```python
from build123d import *

# Parameters (mm, degrees)
F0_W     = 120
F0_H     = 80
F1_DEPTH = 45
F2_R     = 8
F3_T     = -3
F5_DEPTH = 1.5


with BuildPart() as f1:
    # F0 (on Front) → F1 (new body, symmetric)
    with BuildSketch(Plane.XZ):
        Rectangle(F0_W, F0_H)
    extrude(amount=F1_DEPTH, both=True)

    # F2
    f2_edges = [f1.edges().sort_by_distance(p)[0] for p in [
        (60, 0, 40),
        (60, -45, 0),
        (60, 45, 0),
        (-60, 45, 0),
        (0, 45, 40),
        (-60, 0, 40),
        (-60, -45, 0),
        (0, -45, 40),
    ]]
    fillet(f2_edges, radius=F2_R)

    # F3
    f3_openings = [f1.faces().sort_by_distance(p)[0] for p in [
        (0, 0, -40),
    ]]
    offset(amount=F3_T, openings=f3_openings)

    # F4 (on face) → F5 (cut)
    with BuildSketch(Plane(origin=(0, 0, -40), x_dir=(1, 0, 0), z_dir=(0, 0, -1))):
        with BuildLine():
            Line((52, 43.2), (-52, 43.2))
            ThreePointArc((-52, 43.2), (-56.3840620434, 41.3840620434), (-58.2, 37))
            Line((-58.2, 37), (-58.2, -37))
            ThreePointArc((-58.2, -37), (-56.3840620434, -41.3840620434), (-52, -43.2))
            Line((-52, -43.2), (52, -43.2))
            ThreePointArc((52, -43.2), (56.3840620434, -41.3840620434), (58.2, -37))
            Line((58.2, -37), (58.2, 37))
            ThreePointArc((58.2, 37), (56.3840620434, 41.3840620434), (52, 43.2))
        make_face()
    extrude(amount=-F5_DEPTH, mode=Mode.SUBTRACT)


solid = f1.part
```
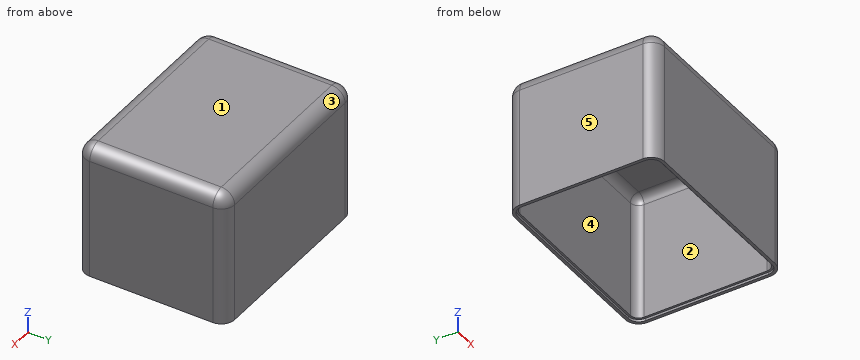
Read the model definition and answer for the solid it produces. Units are mm, in the model's axes. Face numbers are marked on the shaded views. A direction names the side the tool comes from. Give positions to 0.01 mm unless a question says otherwise; leave off trailing zeros. Write each loop counter-clockwise with the first axis right and the second up, starting at its lowest first coordinate (ties: lowest second). Pieces come first, ordered by that corner, then holes. Notation, with made-up numbers: M 23.5,51.25 L 40.5,51.25 A19 cw 40.5,65.25 Z; hole C -2.75,59.25 d6. An arc over 180 degrees is marked long. Put each result on its own line as item: value. Start each with the question number.
1. The part is cut by section B-B, the plane x = 32.5. Give the vertices of the cut face in (y, z), and give its area (3 significant figures).
2. Which of the six approach directions +Z, -Z, +X, -X, +Y, -Y give full straight-line access (tool end or side, diameter ignored) to the marked faces 4 and 5?
3. This flat-tipped pin is pushed along its axis until it touches: pin 1 Ø12 at (x, y) = (32, -23) entering from -Z. Where does it stop, or does it pass through?
4. For a pull along Y with two mould halves and no side action, classify the marked faces 1, 2 and 3 as released by +Y, released by -Y, zero draft, split by the parting line, or undercut.
5. Consider line 1 along Y through (x, z) = (-13.5, 9.5); line 2 along X through (y, z) = (-27.5, 24.5); line 3 along Z through (x, y) = (-51, 14). Determine where each line is inside the solid, lowest interval first.
6. The part is cut by section A-A, the plane z = -13. Give the vertices of the cut face in (x, y), and give its area (3 significant figures).
7. The part is cut by section C-C, the plane y = 25.5. Give the vertices of the cut face in (x, z), and give its area (3 significant figures).
Final values:
1. outline: M -45,-40 L -43.2,-40 L -43.2,-38.5 L -42,-38.5 L -42,32 A5 cw -37,37 L 37,37 A5 cw 42,32 L 42,-38.5 L 43.2,-38.5 L 43.2,-40 L 45,-40 L 45,32 A8 ccw 37,40 L -37,40 A8 ccw -45,32 Z
1. area: 712 mm²
2. face 4: -Z
2. face 5: +Z, -Z, -X, +Y, -Y
3. pin 1: stops at z = 37
4. face 1: zero draft
4. face 2: undercut
4. face 3: released by +Y
5. line 1: y = -45 to -42, 42 to 45
5. line 2: x = -60 to -57, 57 to 60
5. line 3: z = 37 to 40
6. outline: M -60,-37 A8 ccw -52,-45 L 52,-45 A8 ccw 60,-37 L 60,37 A8 ccw 52,45 L -52,45 A8 ccw -60,37 Z; hole M -57,-37 A5 ccw -52,-42 L 52,-42 A5 ccw 57,-37 L 57,37 A5 ccw 52,42 L -52,42 A5 ccw -57,37 Z
6. area: 1,190 mm²
7. outline: M -60,-40 L -58.2,-40 L -58.2,-38.5 L -57,-38.5 L -57,32 A5 cw -52,37 L 52,37 A5 cw 57,32 L 57,-38.5 L 58.2,-38.5 L 58.2,-40 L 60,-40 L 60,32 A8 ccw 52,40 L -52,40 A8 ccw -60,32 Z
7. area: 802 mm²
